Part model, mm, in its own coordinate system. A direction names the side the tool comes from. Round coordinates to 2 decimals unless told otherwise and drop trailing zeros. Loops run counter-clockwise (first coordinate to the right, second up) from the corner with the lowest first, then second, coordinate; pieces in that order, holes last.
1) Mould opens along Y. For faces 3 (the flat face through (32, 40, -41)), 4 (the flat face through (0, 20, -33)), 5 (the flat face through (42, 0, -33)) say: +Y half, -Y half, draft (parallel to the pull), parting line (faces both ways), or undercut.
2) Probe line 1 (Y direction, x = 79, z = -11); line 2 (X direction, y = 12, z = -10); line 3 (X direction, y = 24.5, z = -15). List the from-to ranges inside material, lowest first.
3) 3-axis set-ups, long thin cutter, end or side, ignore diameter. For faces 1 (the flat face through (73, 28, -30)), 2 (the flat face through (42, 20, -66)): which of +Z, -Z, +X, -X, +Y, -Y reach the whole face in a straight line?
4) Band-saw the part on C-C, the plane y = 36.5. Write the cut outline in (x, z).
5) Drop a flat-ended pin along its axis: P1, Ø5, axis at x = 74, z = -25, coming from the +Y side. Give the stop position or say it passes through.
from build123d import *

# Parameters (mm, degrees)
SKETCH1_W               = 85
SKETCH1_H               = 66
BOSS_EXTRUDE1_DEPTH     = 40
CUT_EXTRUDE1_DEPTH      = 115.808536268
CUT_EXTRUDE1_DEPTH_BACK = 30
CHAMFER1_SIZE2          = 20
CHAMFER1_SIZE           = 30


with BuildPart() as part:
    # Sketch1 → Boss-Extrude1 (new body)
    with BuildSketch(Plane(origin=(0, 0, 0), x_dir=(1, 0, 0), z_dir=(0, 1, 0))):
        with Locations((42.5, 33)):
            Rectangle(SKETCH1_W, SKETCH1_H)
    extrude(amount=BOSS_EXTRUDE1_DEPTH)

    # Sketch3 → Cut-Extrude1 (cut, two sides: drawn at the far end of the back side and taken through both)
    with BuildSketch(Plane(origin=(0, 40, 0), x_dir=(1, 0, 0), z_dir=(0, 1, 0)).offset(-CUT_EXTRUDE1_DEPTH_BACK)):
        Polygon((280.267374354, 30), (85, 30), (75, 30), (65, 0), (3.251034432, -185.246896704), (242.87031101, -493.629763025), (519.886650932, -278.382866321), align=None)
    extrude(amount=CUT_EXTRUDE1_DEPTH + CUT_EXTRUDE1_DEPTH_BACK, mode=Mode.SUBTRACT)

    # Chamfer1
    chamfer1_edges = [part.edges().sort_by_distance(p)[0] for p in [
        (70, 40, -15),
    ]]
    chamfer1_side = [part.faces().sort_by_distance(p)[0] for p in [
        (70, 39.6, -15),
    ]]
    chamfer(chamfer1_edges, length=CHAMFER1_SIZE - 0.0001, length2=CHAMFER1_SIZE2 - 0.0001, reference=chamfer1_side[0])  # a hair under: the kernel refuses the full size


solid = part.part
Reported:
1. face 3: +Y half
1. face 4: draft
1. face 5: -Y half
2. line 1: y = 0 to 10
2. line 2: x = 0 to 66.93
2. line 3: x = 0 to 59.81
3. face 1: +Z, +X, +Y
3. face 2: -Z, +X, -X, +Y, -Y
4. outline: (0, -66) - (85, -66) - (85, -30) - (56.38, -30) - (46.38, 0) - (0, 0) - close
5. P1: stops at y = 12.8
